from build123d import *

# Parameters (mm, degrees)
F0_W           = 300
F0_H           = 200
F1_DEPTH       = 40
F2_R           = 15.75
F2_R_2         = 15.748
F3_DEPTH       = 20
F4_R           = 8.75
F4_R_2         = 8.7503
F5_DEPTH       = 40.001
F6_W           = 40
F6_H           = 200
F7_DEPTH       = 260
F8_R           = 50
F9_DEPTH       = 300.001
F11_D          = 12.1
F12_SIZE       = 10
F14_DEPTH      = 25
F14_DEPTH_BACK = 25


with BuildPart() as f1:
    # F0 (on Top) → F1 (new body)
    with BuildSketch(Plane.XY):
        with Locations((-9.0769985841, 3.5027405247)):
            Rectangle(F0_W, F0_H)
    extrude(amount=F1_DEPTH)

    # F2 (on face) → F3 (cut)
    with BuildSketch(Plane.XY.offset(40)):
        with Locations((100.9230014159, 63.5027405247)):
            Circle(F2_R)
        with Locations((100.9230014159, -56.4972594753)):
            Circle(F2_R)
        with Locations((-19.0769985841, 63.4977405247)):
            Circle(F2_R_2)
        with Locations((-19.0769985841, -56.4922594753)):
            Circle(F2_R_2)
    extrude(amount=-F3_DEPTH, mode=Mode.SUBTRACT)

    # F4 (on face) → F5 (cut, through all)
    with BuildSketch(Plane.XY.offset(40)):
        with Locations((-19.0769985841, 63.4977405247)):
            Circle(F4_R)
        with Locations((100.9230014159, 63.5027405247)):
            Circle(F4_R_2)
        with Locations((-19.0769985841, -56.4922594753)):
            Circle(F4_R_2)
        with Locations((100.9230014159, -56.4972594753)):
            Circle(F4_R_2)
    extrude(amount=-F5_DEPTH, mode=Mode.SUBTRACT)

    # F6 (on face) → F7 (join)
    with BuildSketch(Plane.XY.offset(40)):
        with Locations((-139.0769985841, 3.5027405247)):
            Rectangle(F6_W, F6_H)
    extrude(amount=F7_DEPTH)

    # F8 (on face) → F9 (cut, through all)
    with BuildSketch(Plane(origin=(-159.0769985841, 0, 0), x_dir=(0, -1, 0), z_dir=(-1, 0, 0))):
        with Locations((-3.5027405247, 200)):
            Circle(F8_R)
        with BuildLine():
            ThreePointArc((-3.5027399336, 300), (67.2079378029, 270.7106779097), (96.4972594753, 200))
            Line((96.4972594753, 200), (96.4972594753, 300))
            Line((96.4972594753, 300), (-3.5027399336, 300))
        make_face()
        with BuildLine():
            ThreePointArc((-103.5027405247, 200), (-74.2134184344, 270.7106783276), (-3.5027399336, 300))
            Line((-3.5027399336, 300), (-103.5027405247, 300))
            Line((-103.5027405247, 300), (-103.5027405247, 200))
        make_face()
    extrude(amount=-F9_DEPTH, mode=Mode.SUBTRACT)

    # F11 (through all)
    with Locations(Plane.YZ.offset(-119.0769985841)):
        with Locations((3.5027405247, 272), (75.5027405247, 200), (3.5027405247, 128), (-68.4972594753, 200)):
            Hole(F11_D / 2)

    # F12
    f12_edges = [f1.edges().sort_by_distance(p)[0] for p in [
        (140.923001, -96.497259, 20),
        (140.923001, 103.502741, 20),
        (-159.076999, 3.502741, 0),
    ]]
    chamfer(f12_edges, length=F12_SIZE)

    # F13 (on Front) → F14 (join, two sides)
    with BuildSketch(Plane.XZ) as f14_sk:
        Polygon((-119.0769985841, 100), (-119.0769985841, 40), (-57.3225580156, 40), align=None)
    extrude(amount=F14_DEPTH)
    extrude(f14_sk.sketch, amount=-F14_DEPTH_BACK)


solid = f1.part
The listing builds one solid part. Answer for the finished solid, in the listing's coordinates (mm). A direction names the side the tool comes from. Give positions to 0.01 mm unless a question says otherwise; leave off trailing zeros. Order: outer loops, then holes, each group sorted by start corner. A loop starts at its lowest first (then second) coordinate and runs counter-clockwise, first axis right, second up. Notation, with made-up numbers: (15, 18.5) - (28, 18.5) arc R21 cw to (28, 56.5) - close; hole circle Ø5 at (86.25, 61.25). An arc over 180 degrees is marked (long way). One line per item, written item: value. Start each with the question number.
1) The mould has two halves that part along Y. Classify faces 1 (the face through (-21.13, -40.88, 30.14)), 2 (the face through (135.99, -91.43, 19.72)), 3 (the face through (-102, 25, 57)), 4 (the face through (140.923, 2, 20)): released by +Y, released by -Y, zero draft, split by the parting line, or undercut.
2) Find the intervals of material crossed by L1, parallel to X at y = 32, z = 242; L2, parallel to Z at x = -35, y = 73; L3, parallel to Z at x = 93, y = 68, in increasing order.
3) Given pin 1 Ø7.5 at (y, z) = (-68.5, 200) entering from -X; pin 2 Ø2 at (y, z) = (-74, 87.5) entering from +X; pin 3 Ø25 at (x, y) = (97.5, 58) entering from +Z; pin 4 Ø9.5 at (x, y) = (-18, -50.5) entering from +Z, each flat-ended and moving along its own axis, determine where each tip first touches the part or whether it passes through.
4) A cutting plane is placed at A-A on y = 3.5. Give the vertices of the cut face in (x, z).
5) A tool of negligible diameter and unlimited length cuts with its end or side. For faces 5 (the face through (-30.684, 74.141, 30.14)), 6 (the face through (135.993, 98.433, 19.72)), 7 (the face through (-102, -25, 57)), from which of +Z, -Z, +X, -X, +Y, -Y can it reach the whole face along a straight path? Write none if from no direction.
6) A cutting plane is placed at C-C on y = -34. Give the vertices of the cut face in (x, z).
7) A cutting plane is placed at D-D on x = -79. Give the vertices of the cut face in (y, z), then the cut area to 3 significant figures.
8) A cutting plane is placed at B-B on z = 128. Give the vertices of the cut face in (x, y).
Answer sheet:
1. face 1: undercut
1. face 2: released by -Y
1. face 3: released by +Y
1. face 4: zero draft
2. L1: x = -159.08 to -119.08
2. L2: z = 0 to 40
2. L3: z = 0 to 20
3. pin 1: passes through
3. pin 2: stops at x = -119.08
3. pin 3: stops at z = 40
3. pin 4: stops at z = 20
4. outline: (-159.08, 10) - (-149.08, 0) - (140.92, 0) - (140.92, 40) - (-57.32, 40) - (-119.08, 100) - (-119.08, 121.95) - (-159.08, 121.95) - close; (-159.08, 134.05) - (-119.08, 134.05) - (-119.08, 150) - (-159.08, 150) - close; (-159.08, 250) - (-119.08, 250) - (-119.08, 265.95) - (-159.08, 265.95) - close; (-159.08, 278.05) - (-119.08, 278.05) - (-119.08, 300) - (-159.08, 300) - close
5. face 5: +Z
5. face 6: +Z, -Z, +X, +Y
5. face 7: +Z, +X, -Y
6. outline: (-159.08, 10) - (-149.08, 0) - (140.92, 0) - (140.92, 40) - (-119.08, 40) - (-119.08, 166.93) - (-159.08, 166.93) - close; (-159.08, 233.07) - (-119.08, 233.07) - (-119.08, 292.7) - (-159.08, 292.7) - close
7. outline: (-96.5, 0) - (103.5, 0) - (103.5, 40) - (25, 40) - (25, 61.06) - (-25, 61.06) - (-25, 40) - (-96.5, 40) - close
7. area: 9,050 mm2
8. outline: (-159.08, -96.5) - (-119.08, -96.5) - (-119.08, -2.55) - (-159.08, -2.55) - close; (-159.08, 9.55) - (-119.08, 9.55) - (-119.08, 103.5) - (-159.08, 103.5) - close
